Verification items for the finished model (mm, model axes). Round coordinates to 2 decimals unless told otherwise and drop trailing zeros. Order: outer loops, then holes, each group sorted by start corner. A loop starts at its lowest first (then second) coordinate and runs counter-clockwise, first axis right, second up. Notation, with made-up numbers: M -8.75,-25 L 3.25,-25 A8 cw 3.25,-15 Z; hole C -13,-18.75 d1. An arc over 180 degrees is marked long. Use CSV: the item, a comma, the result in double quotes. Start each with the question number.
Q1. Sectioned sample at C-C (z = 2.55). State how many separate pieces and enclosed holes the cut face has, and give its area (3 significant figures).
Q2. Gauge pin test, flat ends, axial feed: pin 1 Ø2.5 at (x, y) = (47.25, 54.32) entering from -Z; pin 2 Ø3.5 at (x, y) = (59.25, -6.46) entering from +Z. Record the tip position at first contact, or that the pin passes through.
Q3. Scan lines: line 1 (X direction, y = 37.5, z = 2.8); line 2 (X direction, y = -41, z = 0.35); line 3 (X direction, y = 5.5, z = 2.15). Record each from-to range of solid material in increasing order.
Q4. Sectioned sample at B-B (x = 30). Enter the section's corners in (y, z), and give its area (3 significant figures).
Q5. Sectioned sample at A-A (x = 13). Enter the section's corners in (y, z), and give its area (3 significant figures).
```python
from build123d import *

# Parameters (mm, degrees)
SKETCH4_R           = 1.54999944
SKETCH4_R_2         = 1.6
SKETCH4_R_3         = 2.6
BOSS_EXTRUDE6_DEPTH = 3


with BuildPart() as part:
    # Sketch4 → Boss-Extrude6 (new body)
    with BuildSketch(Plane.XY):
        with BuildLine():
            Line((50.251854725, 14.295018861), (50.251854725, 57.295018861))
            Line((50.251854725, 57.295018861), (-44.769148998, 57.295018861))
            Line((-44.769148998, 57.295018861), (-44.769148998, 14.295018861))
            ThreePointArc((-44.769148998, 14.295018861), (-45.354935436, 12.880805298), (-46.769148998, 12.295018861))
            Line((-46.769148998, 12.295018861), (-57.769148998, 12.295018861))
            ThreePointArc((-57.769148998, 12.295018861), (-59.183362561, 11.709232423), (-59.769148998, 10.295018861))
            Line((-59.769148998, 10.295018861), (-59.769148998, -10.71398001))
            ThreePointArc((-59.769148998, -10.71398001), (-59.183362561, -12.128193573), (-57.769148998, -12.71398001))
            Line((-57.769148998, -12.71398001), (-46.769148998, -12.71398001))
            ThreePointArc((-46.769148998, -12.71398001), (-45.354935436, -13.299766448), (-44.769148998, -14.71398001))
            Line((-44.769148998, -14.71398001), (-44.769148998, -57.71398001))
            Line((-44.769148998, -57.71398001), (50.251854725, -57.71398001))
            Line((50.251854725, -57.71398001), (50.251854725, -14.71398001))
            ThreePointArc((50.251854725, -14.71398001), (50.837641163, -13.299766448), (52.251854725, -12.71398001))
            Line((52.251854725, -12.71398001), (63.251854725, -12.71398001))
            ThreePointArc((63.251854725, -12.71398001), (64.666068287, -12.128193573), (65.251854725, -10.71398001))
            Line((65.251854725, -10.71398001), (65.251854725, 10.295018861))
            ThreePointArc((65.251854725, 10.295018861), (64.666068287, 11.709232423), (63.251854725, 12.295018861))
            Line((63.251854725, 12.295018861), (52.251854725, 12.295018861))
            ThreePointArc((52.251854725, 12.295018861), (50.837641163, 12.880805298), (50.251854725, 14.295018861))
        make_face()
        with Locations((47.251855645, 15.295019041)):
            Circle(SKETCH4_R, mode=Mode.SUBTRACT)
        with Locations((2.741352863, 54.315928454)):
            Circle(SKETCH4_R, mode=Mode.SUBTRACT)
        with Locations((-31.748146375, 15.295019041)):
            Circle(SKETCH4_R, mode=Mode.SUBTRACT)
        with Locations((-41.769148998, -0.71398001)):
            Circle(SKETCH4_R_2, mode=Mode.SUBTRACT)
        with Locations((47.251854725, -0.71398001)):
            Circle(SKETCH4_R_2, mode=Mode.SUBTRACT)
        with Locations((-41.769148998, -54.71398001)):
            Circle(SKETCH4_R_2, mode=Mode.SUBTRACT)
        with Locations((47.251854725, -54.71398001)):
            Circle(SKETCH4_R_2, mode=Mode.SUBTRACT)
        with Locations((-39.969148998, -5.97675003)):
            Circle(SKETCH4_R_2, mode=Mode.SUBTRACT)
        with Locations((-39.969148998, -27.618447294)):
            Circle(SKETCH4_R_2, mode=Mode.SUBTRACT)
        with Locations((-39.969148998, -49.451209991)):
            Circle(SKETCH4_R_2, mode=Mode.SUBTRACT)
        with Locations((59.251854725, -0.209480575)):
            Circle(SKETCH4_R_3, mode=Mode.SUBTRACT)
        with Locations((-41.769148998, 54.315928454)):
            Circle(SKETCH4_R_2, mode=Mode.SUBTRACT)
        with Locations((47.251855645, 54.315928454)):
            Circle(SKETCH4_R_2, mode=Mode.SUBTRACT)
        with Locations((59.251854725, 6.042769143)):
            Circle(SKETCH4_R_2, mode=Mode.SUBTRACT)
        with Locations((59.251854725, -6.461730293)):
            Circle(SKETCH4_R_2, mode=Mode.SUBTRACT)
        with Locations((-53.769148998, -0.209480575)):
            Circle(SKETCH4_R_3, mode=Mode.SUBTRACT)
        with Locations((-53.769148998, 6.042769143)):
            Circle(SKETCH4_R_2, mode=Mode.SUBTRACT)
        with Locations((-53.769148998, -6.461730293)):
            Circle(SKETCH4_R_2, mode=Mode.SUBTRACT)
        with BuildLine():
            Line((-12.258647137, 43.865161879), (17.741352863, 43.865161879))
            ThreePointArc((17.741352863, 43.865161879), (20.741352863, 40.865161879), (17.741352863, 37.865161879))
            Line((17.741352863, 37.865161879), (-12.258647137, 37.865161879))
            ThreePointArc((-12.258647137, 37.865161879), (-15.258647137, 40.865161879), (-12.258647137, 43.865161879))
        make_face(mode=Mode.SUBTRACT)
        with BuildLine():
            Line((-12.258647137, 27.435304897), (17.741352863, 27.435304897))
            ThreePointArc((17.741352863, 27.435304897), (20.741352863, 24.435304897), (17.741352863, 21.435304897))
            Line((17.741352863, 21.435304897), (-12.258647137, 21.435304897))
            ThreePointArc((-12.258647137, 21.435304897), (-15.258647137, 24.435304897), (-12.258647137, 27.435304897))
        make_face(mode=Mode.SUBTRACT)
        with BuildLine():
            Line((-12.258647137, 11.005447916), (17.741352863, 11.005447916))
            ThreePointArc((17.741352863, 11.005447916), (20.741352863, 8.005447916), (17.741352863, 5.005447916))
            Line((17.741352863, 5.005447916), (-12.258647137, 5.005447916))
            ThreePointArc((-12.258647137, 5.005447916), (-15.258647137, 8.005447916), (-12.258647137, 11.005447916))
        make_face(mode=Mode.SUBTRACT)
        with BuildLine():
            Line((-12.258647137, -5.424409066), (17.741352863, -5.424409066))
            ThreePointArc((17.741352863, -5.424409066), (20.741352863, -8.424409066), (17.741352863, -11.424409066))
            Line((17.741352863, -11.424409066), (-12.258647137, -11.424409066))
            ThreePointArc((-12.258647137, -11.424409066), (-15.258647137, -8.424409066), (-12.258647137, -5.424409066))
        make_face(mode=Mode.SUBTRACT)
        with BuildLine():
            Line((-12.258647137, -21.854266047), (17.741352863, -21.854266047))
            ThreePointArc((17.741352863, -21.854266047), (20.741352863, -24.854266047), (17.741352863, -27.854266047))
            Line((17.741352863, -27.854266047), (-12.258647137, -27.854266047))
            ThreePointArc((-12.258647137, -27.854266047), (-15.258647137, -24.854266047), (-12.258647137, -21.854266047))
        make_face(mode=Mode.SUBTRACT)
        with BuildLine():
            Line((-12.258647137, -38.284123029), (17.741352863, -38.284123029))
            ThreePointArc((17.741352863, -38.284123029), (20.741352863, -41.284123029), (17.741352863, -44.284123029))
            Line((17.741352863, -44.284123029), (-12.258647137, -44.284123029))
            ThreePointArc((-12.258647137, -44.284123029), (-15.258647137, -41.284123029), (-12.258647137, -38.284123029))
        make_face(mode=Mode.SUBTRACT)
        with BuildLine():
            Line((-20.769148998, 37.295018861), (-20.769148998, -37.71398001))
            ThreePointArc((-20.769148998, -37.71398001), (-23.769148998, -40.71398001), (-26.769148998, -37.71398001))
            Line((-26.769148998, -37.71398001), (-26.769148998, 37.295018861))
            ThreePointArc((-26.769148998, 37.295018861), (-23.769148998, 40.295018861), (-20.769148998, 37.295018861))
        make_face(mode=Mode.SUBTRACT)
        with BuildLine():
            Line((32.251854725, 37.295018861), (32.251854725, -37.71398001))
            ThreePointArc((32.251854725, -37.71398001), (29.251854725, -40.71398001), (26.251854725, -37.71398001))
            Line((26.251854725, -37.71398001), (26.251854725, 37.295018861))
            ThreePointArc((26.251854725, 37.295018861), (29.251854725, 40.295018861), (32.251854725, 37.295018861))
        make_face(mode=Mode.SUBTRACT)
    extrude(amount=BOSS_EXTRUDE6_DEPTH)


solid = part.part
```
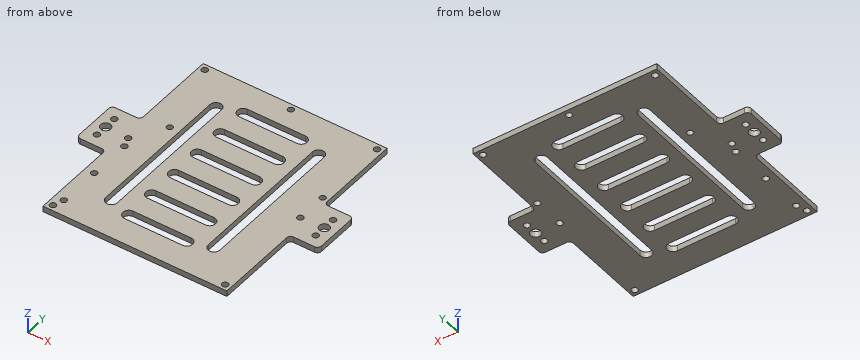
Verdict:
1,separate pieces,"1"
1,enclosed holes,"26"
1,area,"9,300 mm²"
2,pin 1,"passes through"
2,pin 2,"stops at z = 3"
3,line 1,"x = -44.77 to -26.76, -20.78 to 26.26, 32.24 to 50.25"
3,line 2,"x = -44.77 to -15.25, 20.73 to 50.25"
3,line 3,"x = -59.77 to -55.27, -52.26 to -26.77, -20.77 to -13.91, 19.39 to 26.25, 32.25 to 57.75, 60.76 to 65.25"
4,outline,"M -57.71,0 L -40.62,0 L -40.62,3 L -57.71,3 Z; M 40.2,0 L 57.3,0 L 57.3,3 L 40.2,3 Z"
4,area,"103 mm²"
5,outline,"M -57.71,0 L -44.28,0 L -44.28,3 L -57.71,3 Z; M -38.28,0 L -27.85,0 L -27.85,3 L -38.28,3 Z; M -21.85,0 L -11.42,0 L -11.42,3 L -21.85,3 Z; M -5.42,0 L 5.01,0 L 5.01,3 L -5.42,3 Z; M 11.01,0 L 21.44,0 L 21.44,3 L 11.01,3 Z; M 27.44,0 L 37.87,0 L 37.87,3 L 27.44,3 Z; M 43.87,0 L 57.3,0 L 57.3,3 L 43.87,3 Z"
5,area,"237 mm²"
